Autodesk Inventor part; units mm, degrees
ref_plane "YZ Plane" through (0, 0, 0) normal (1, 0, 0) x (0, 1, 0)
ref_plane "XZ Plane" through (0, 0, 0) normal (0, 1, 0) x (-1, 0, 0)
ref_plane "XY Plane" through (0, 0, 0) normal (0, 0, 1) x (1, 0, 0)
sketch "草圖1" plane through (0, 0, 0) normal (0, 0, 1) x (1, 0, 0)
  line L0 (0, 0) -> (13.2614, 34.1988)
  line L1 (11.3356, 23.643) -> (10.4709, 21.8396)
  line L2 (11.3967, 34.9219) -> (-1.8647, 0.7231)
  line L3 (13.255, 23.0202) -> (1.8034, -0.8647)
  line L4 (13.2272, 22.8679) -> (15.2289, 33.8398)
  arc A0 (13.139, 22.7784) -> (13.3031, 23.2841) centre (11.3356, 23.643) ccw
  arc A1 (15.2289, 33.8398) -> (11.3967, 34.9219) centre (13.2614, 34.1988) ccw
  arc A2 (12.5383, 32.3341) -> (12.9025, 32.2313) centre (13.2614, 34.1988) ccw
  arc A3 (0.8647, 1.8034) -> (0.7231, 1.8647) centre (0, 0) ccw
  arc A4 (-1.8647, 0.7231) -> (1.8034, -0.8647) centre (0, 0) ccw
  dimension "d0" = 10.73
  dimension "d1" = 26.22
  dimension "d2" = 36.68
extrude "擠出1" add sketch "草圖1" along normal blind 1 contours A1 L4 A0 L3 A4 L2
sketch "草圖2" plane through (0, 0, 1) normal (0, 0, 1) x (1, 0, 0)
  arc A0 (13.139, 22.7784) -> (13.3031, 23.2841) centre (11.3356, 23.643) ccw
  circle A1 centre (11.3356, 23.643) radius 1
  arc A2 (15.2289, 33.8398) -> (11.3967, 34.9219) centre (13.2614, 34.1988) ccw
  circle A3 centre (13.2614, 34.1988) radius 1
  arc A4 (-1.8647, 0.7231) -> (1.8034, -0.8647) centre (0, 0) ccw
  circle A5 centre (0, 0) radius 1
  dimension "d8" = 2
  dimension "d9" = 2
  dimension "d10" = 2
extrude "擠出2" cut sketch "草圖2" against normal blind 10
properties part number "三角塊3"
Check sheet for the modelled part. Datum: model origin and axes. Units: mm. Round coordinates to 2 decimals unless told otherwise and drop trailing zeros. Loops run counter-clockwise (first coordinate to the right, second up) from the corner with the lowest first, then second, coordinate; pieces in that order, holes last.
1. Sectioned sample at A-A on x = 0. Record the boundary of the cut face in (y, z).
2. Sectioned sample at B-B on y = 0. Record the boundary of the cut face in (x, z).
3. Mould release check, pull along Y, two halves, no side actions. Record for faces 1 (the flat face through (14.253, 28.488, 0.493)), 2 (the cylindrical face through (-0.217, -0.976, 0.507)), 3 (the flat face through (4.86, 18.06, 0.49)), 4 (the flat face through (7, 17, 1)): released by +Y, released by -Y, zero draft, split by the parting line, or undercut.
4. Scan lines: probe 1 along Y at (x, z) = (12, 0.7); probe 2 along Y at (x, z) = (11.5, 0.95); probe 3 along X at (y, z) = (11, 0.65). Record each from-to range of solid material in increasing order.
5. Sectioned sample at C-C on z = 0.5. Record the boundary of the cut face in (x, y).
6. Sectioned sample at D-D on y = 27. Record the boundary of the cut face in (x, z), and give its area (3 significant figures).
7. Gauge pin test, flat end, axial feed: pin 1 Ø1.2 at (x, y) = (0, 0) entering from +Z. Record the tip position at first contact, or that the pin passes through.
Recorded:
1. outline: (-2, 0) - (-1, 0) - (-1, 1) - (-2, 1) - close; (1, 0) - (5.53, 0) - (5.53, 1) - (1, 1) - close
2. outline: (-2, 0) - (-1, 0) - (-1, 1) - (-2, 1) - close; (1, 0) - (2.22, 0) - (2.22, 1) - (1, 1) - close
3. face 1: released by -Y
3. face 2: undercut
3. face 3: released by +Y
3. face 4: zero draft
4. probe 1: y = 20.4 to 22.9, 24.39 to 35.75
4. probe 2: y = 19.36 to 22.66, 24.63 to 35.15
4. probe 3: x = 2.12 to 7.49
5. outline: (-1.86, 0.72) arc R2 ccw to (1.8, -0.86) - (13.14, 22.78) arc R2 ccw to (13.3, 23.28) - (15.23, 33.84) arc R2 ccw to (11.4, 34.92) - close; hole circle Ø2 at (0, 0); hole circle Ø2 at (11.34, 23.64); hole circle Ø2 at (13.26, 34.2)
6. outline: (8.32, 0) - (13.98, 0) - (13.98, 1) - (8.32, 1) - close
6. area: 5.66 mm2
7. pin 1: passes through
